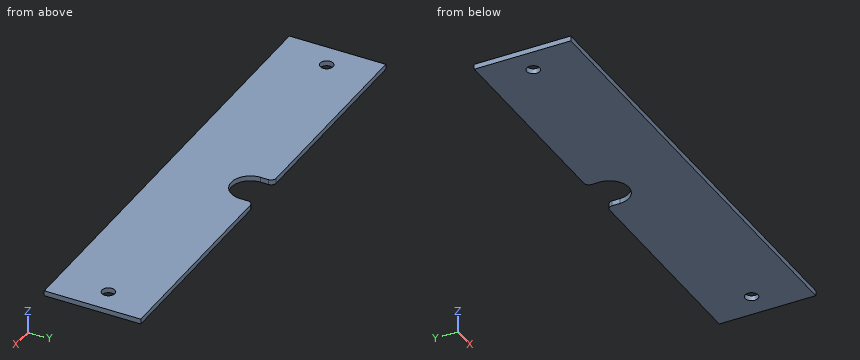
from build123d import *

# Parameters (mm, degrees)
ESQUISSE1_R        = 2.5
BOSS_EXTRU_1_DEPTH = 2
CONG_1_R           = 2


with BuildPart() as part:
    # Esquisse1 → Boss.-Extru.1 (new body)
    with BuildSketch(Plane.XY):
        with BuildLine():
            Line((-89.8, 18.8), (-89.8, -18.8))
            Line((-89.8, -18.8), (89.8, -18.8))
            Line((89.8, -18.8), (89.8, 18.8))
            Line((89.8, 18.8), (7.5, 18.8))
            Line((7.5, 18.8), (7.5, 13.8))
            ThreePointArc((7.5, 13.8), (0, 6.3), (-7.5, 13.8))
            Line((-7.5, 13.8), (-7.5, 18.8))
            Line((-7.5, 18.8), (-89.8, 18.8))
        make_face()
        with Locations((-80, 1)):
            Circle(ESQUISSE1_R, mode=Mode.SUBTRACT)
        with Locations((80, 1)):
            Circle(ESQUISSE1_R, mode=Mode.SUBTRACT)
    extrude(amount=BOSS_EXTRU_1_DEPTH)

    # Congé1
    cong_1_edges = [part.edges().sort_by_distance(p)[0] for p in [
        (7.5, 18.8, 1),
        (-7.5, 18.8, 1),
    ]]
    fillet(cong_1_edges, radius=CONG_1_R)


solid = part.part
Could you check a few things on this model? Use its own coordinates, in mm. Round coordinates to 2 decimals unless told otherwise and drop trailing zeros. Loops run counter-clockwise (first coordinate to the right, second up) from the corner with the lowest first, then second, coordinate; pieces in that order, holes last. Notation, with made-up numbers: (34.5, 23) - (87.5, 23) arc R21 cw to (87.5, 30) - close; hole circle Ø11 at (1.25, -8.5). An arc over 180 degrees is marked (long way). Write item = value, one per line.
1) I need wall thicknesses on line 1 along Y through (x, z) = (-80, 0.7); line 2 along X through (y, z) = (-0.5, 1.4); line 3 along X through (y, z) = (13, 0.95). Which ranges of each line are inside material? Lowest first, please. Write a range as from..to.
Computed:
line_1 = -18.8..-1.5, 3.5..18.8
line_2 = -89.8..-82, -78..78, 82..89.8
line_3 = -89.8..-7.46, 7.46..89.8
2) Imagine slicing it at D-D (y = 12). Please give me the cut outline in (x, z), and give its area (3 significant figures).
Computed:
outline = (-89.8, 0) - (-7.28, 0) - (-7.28, 2) - (-89.8, 2) - close; (7.28, 0) - (89.8, 0) - (89.8, 2) - (7.28, 2) - close
area = 330 mm2
3) Imagine slicing it at C-C (z = 0.95). Please give me the cut outline in (x, y).
Computed:
outline = (-89.8, -18.8) - (89.8, -18.8) - (89.8, 18.8) - (9.5, 18.8) arc R2 ccw to (7.5, 16.8) - (7.5, 13.8) arc R7.5 cw to (-7.5, 13.8) - (-7.5, 16.8) arc R2 ccw to (-9.5, 18.8) - (-89.8, 18.8) - close; hole circle Ø5 at (-80, 1); hole circle Ø5 at (80, 1)
4) Imagine slicing it at B-B (y = 1). Please give me the cut outline in (x, z), and give its area (3 significant figures).
Computed:
outline = (-89.8, 0) - (-82.5, 0) - (-82.5, 2) - (-89.8, 2) - close; (-77.5, 0) - (77.5, 0) - (77.5, 2) - (-77.5, 2) - close; (82.5, 0) - (89.8, 0) - (89.8, 2) - (82.5, 2) - close
area = 339 mm2
5) Imagine slicing it at A-A (x = 80). Please give me the cut outline in (y, z), and give its area (3 significant figures).
Computed:
outline = (-18.8, 0) - (-1.5, 0) - (-1.5, 2) - (-18.8, 2) - close; (3.5, 0) - (18.8, 0) - (18.8, 2) - (3.5, 2) - close
area = 65.2 mm2
